from build123d import *

# Parameters (mm, degrees)
BOSS_EXTRUDE1_DEPTH = 2
FILLET2_R           = 1


with BuildPart() as part:
    # Sketch1 → Boss-Extrude1 (new body)
    with BuildSketch(Plane(origin=(0, 0, 0), x_dir=(1, 0, 0), z_dir=(0, 1, 0))):
        Polygon((0, 0), (-20, 0), (-4.977119068, 30), (45.022880932, 30), align=None)
    extrude(amount=BOSS_EXTRUDE1_DEPTH)

    # Fillet2
    fillet2_edges = [part.edges().sort_by_distance(p)[0] for p in [
        (-12.488559534, 2, -15),
        (-12.488559534, 0, -15),
        (20.022880932, 0, -30),
        (-20, 1, 0),
        (-4.977119068, 1, -30),
        (45.022880932, 1, -30),
        (20.022880932, 2, -30),
    ]]
    fillet(fillet2_edges, radius=FILLET2_R - 0.0001)  # a hair under: the kernel refuses the full size


solid = part.part
Input: part model. Units: mm. Frame: model coordinates. Give positions to 0.01 mm unless a question says otherwise; leave off trailing zeros. Write each loop counter-clockwise with the first axis right and the second up, starting at its lowest first coordinate (ties: lowest second). Pieces come first, ordered by that corner, then holes. Notation, with made-up numbers: (-8.5, 82) -> (-2.5, 82) arc R32 cw to (-2.5, 117) -> close; hole circle Ø5 at (19, 23.5). An arc over 180 degrees is marked (long way). Use one line per item in the form item = value. Start each with the question number.
1) Section query A-A on y = 0.6. Return the cut outline in (x, z), then the cut area to 3 significant figures.
2) Pin query (flat end, axial travel): pin 1 (1 mm diameter, centred on y = 1, z = -12, fed in from -X); pin 2 (6 mm diameter, centred on x = 25.5, z = -13, fed in from +Y); pin 3 (1 mm diameter, centred on y = 1.5, z = -5.5, fed in from -X). Return the tip coordinate at first contact, or that it passes through.
3) Ray query, probe 1 along Z at (x, y) = (0.5, 0.6); probe 2 along X at (y, z) = (1.8, -26.75); probe 3 along X at (y, z) = (0.3, -5.25). Return the intervals inside material, ascending. Write a range as from..to.
Outcome:
q1.outline = (-19.38, -1.05) -> (-5.18, -29.41) arc R0.92 ccw to (-4.36, -29.92) -> (42.12, -29.92) arc R1 ccw to (42.27, -28.17) -> (0, 0) -> (-18.38, 0) arc R1 ccw to start
q1.area = 1,040 mm^2
q2.pin_1 = -14.24
q2.pin_2 = through
q2.pin_3 = -17.43
q3.probe_1 = -29.92..-0.33
q3.probe_2 = -6.16..40.15
q3.probe_3 = -17.05..7.88
